Input: dimensioned drawing with shaded views. Units: mm. Origin: part minimum x, y, z. A direction names the side the tool comes from. Round coordinates to 2 decimals unless told otherwise and drop trailing zeros. Order: outer loops, then holes, each group sorted by start corner. A loop starts at its lowest first (then second) coordinate and runs counter-clockwise, first axis right, second up. Notation, with made-up numbers: (83.25, 39.25) - (98.25, 39.25) arc R14 cw to (98.25, 51.25) - close; hole circle Ø5 at (70, 32.25). An arc over 180 degrees is marked (long way). Put each result on its own line as item: value. Start each with the question number.
(1) Section A-A (y = 1.55). Output: boundary loops of the cut face in (x, z) (1 decimal).
(2) Pin query (flat end, axial travel): P1, Ø1.5, axis at y = 3.5, z = 4, coming from the -X side; P2, Ø1, axis at y = 0.5, z = 3.5, coming from the +X side; P3, Ø2, axis at x = 7, y = 2.5, coming from the -Z side (1 decimal). Return the tip coordinate at first contact, or that it passes through.
(3) Access query for the marked faces 1 and 2. Directions: +Z, -Z, +X, -X, +Y, -Y. A direction counts if a zero-diameter tool reaches every point of the face in a straight line with its end or side. Return the directions, or none.
(4) Material intervals for L1, parallel to Y at x = 7.5, z = 6; L2, parallel to Z at x = 4.25, y = 1.6 (1 decimal), sorted ascending. Write a range as [from, to].
(5) Section B-B (z = 7.5). Output: boundary loops of the cut face in (x, y).
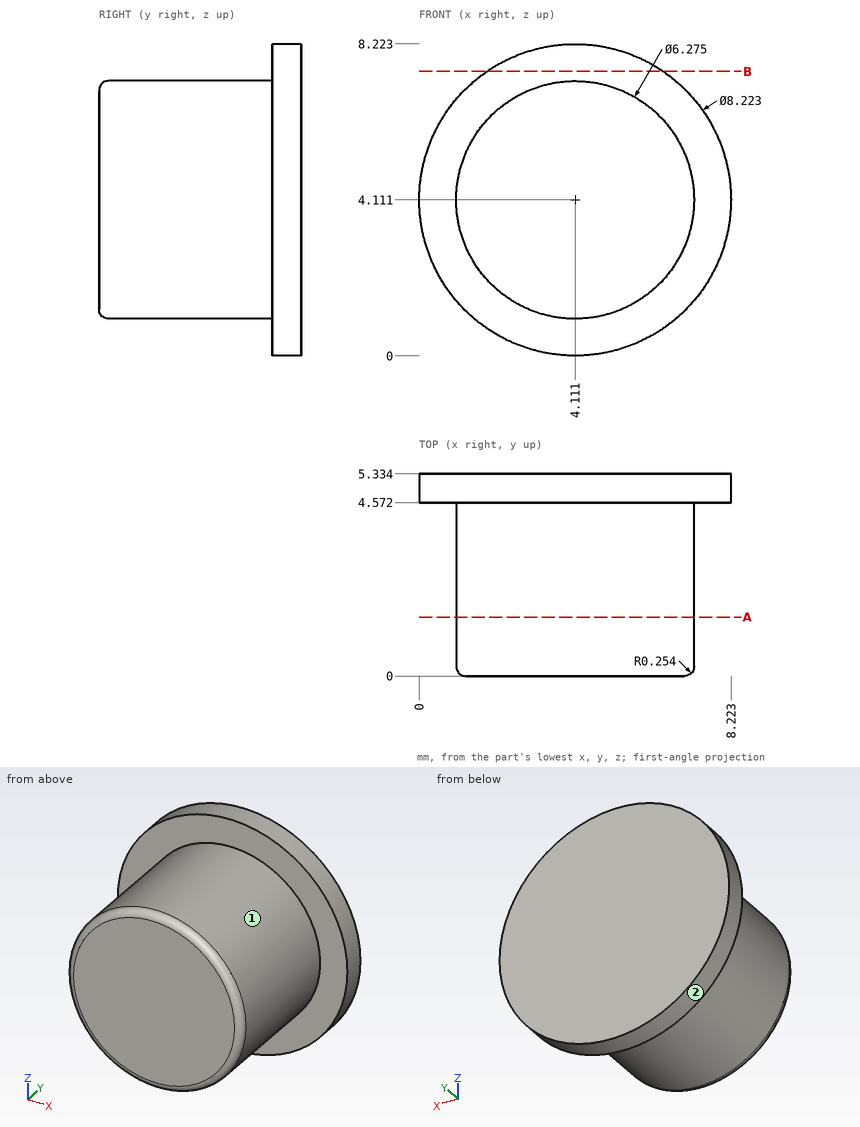
Checks:
1. outline: circle Ø6.3 at (4.1, 4.1)
2. P1: stops at x = 0.97
2. P2: stops at x = 7.25
2. P3: stops at z = 1.6
3. face 1: -Y
3. face 2: +Y, -Y
4. L1: y = [4.57, 5.33]
4. L2: z = [1, 7.2]
5. outline: (1.78, 4.57) - (6.44, 4.57) - (6.44, 5.33) - (1.78, 5.33) - close
